from build123d import *

# Parameters (mm, degrees)
BASE_EXTRUDE_THIN_DEPTH = 142.875
CUT_CNR_DEPTH           = 7.35
CUT_CNR_DEPTH_BACK      = 50.276
HOLE_FLG_D              = 16.764
HOLE_TOP_D              = 13.49375
HOLE_TOP_DEPTH          = 25.4


with BuildPart() as part:
    # Sketch1 → Base-Extrude-Thin (new body)
    with BuildSketch(Plane.XY):
        with BuildLine():
            Line((-228.6, 0), (-6.35, 0))
            ThreePointArc((-6.35, 0), (-1.859871939, -1.859871939), (0, -6.35))
            Line((0, -6.35), (0, -49.276))
            Line((0, -49.276), (6.35, -49.276))
            Line((6.35, -49.276), (6.35, -6.35))
            ThreePointArc((6.35, -6.35), (2.630256121, 2.630256121), (-6.35, 6.35))
            Line((-6.35, 6.35), (-228.6, 6.35))
            Line((-228.6, 6.35), (-228.6, 0))
        make_face()
    extrude(amount=BASE_EXTRUDE_THIN_DEPTH)

    # Sketch2 → Cut cnr (cut, two sides)
    with BuildSketch(Plane(origin=(0, 0, 0), x_dir=(1, 0, 0), z_dir=(0, 1, 0))) as cut_cnr_sk:
        Polygon((-714.082135383, 156.243851855), (-228.6, -50.8), (-12.7, -142.875), (472.782135383, -349.918851855), (58.694431674, -1320.883122621), (-1128.169839092, -814.720418912), align=None)
    extrude(amount=CUT_CNR_DEPTH, mode=Mode.SUBTRACT)
    extrude(cut_cnr_sk.sketch, amount=-CUT_CNR_DEPTH_BACK, mode=Mode.SUBTRACT)

    # Hole-flg (through all)
    with Locations(Plane(origin=(6.35, 0, 0), x_dir=(0, 0, -1), z_dir=(1, 0, 0))):
        with Locations((-120.65, -26.924), (-22.225, -26.924)):
            Hole(HOLE_FLG_D / 2)

    # Hole-top
    with Locations(Plane(origin=(0, 6.35, 0), x_dir=(-1, 0, 0), z_dir=(0, 1, 0))):
        with Locations((203.2, 31.75), (133.35, 31.75)):
            Hole(HOLE_TOP_D / 2, depth=HOLE_TOP_DEPTH)


solid = part.part
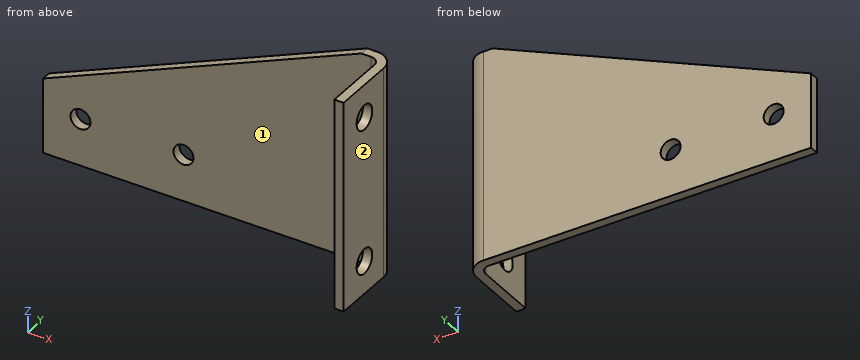
Could you check a few things on this model? Use its own coordinates, in mm. Face numbers are marked on the shaded views. A direction names the side the tool comes from. Coordinates: 2 decimals unless noted, no trailing zeros. Order: outer loops, then holes, each group sorted by start corner. A loop starts at its lowest first (then second) coordinate and runs counter-clockwise, first axis right, second up.
Q1. Suppose I cut it at A-A on x = -133.35. Please give me the cut outline in (y, z).
Q2. Please list where these lines run through material, in increasing order: L1, parallel to Y at x = -34, z = 112.5; L2, parallel to X at y = 3, z = 31.
Q3. Suppose I cut it at D-D on y = -16. Please give me the cut outline in (x, z) (3 decimals), and give its area (3 significant figures).
Q4. Which directions (+Z, -Z, +X, -X, +Y, -Y) give clear straight access to the entire face, cutting with the end or side of a thin tool? Please do the marked faces 1 and 2.
Q5. Suppose I cut it at C-C on z = 41. Please give me the cut outline in (x, y).
Q6. Will these pins go through, and if not, where does the flat tip stop? pin 1 (6 mm diameter, centred on y = -0.5, z = 92, fed in from -X); pin 2 (2 mm diameter, centred on y = -36.5, z = 97.5, fed in from -X); pin 3 (3 mm diameter, centred on y = -1.5, z = 76, fed in from +X); pin 4 (12 mm diameter, centred on x = -203.2, z = 31.75, fed in from +Y).
Q7. Suppose I cut it at B-B on z = 19.5. Please give me the cut outline in (x, y).
Answer:
1. outline: (0, 0) - (6.35, 0) - (6.35, 25) - (0, 25) - close; (0, 38.5) - (6.35, 38.5) - (6.35, 91.42) - (0, 91.42) - close
2. L1: y = 0 to 6.35
2. L2: x = -228.6 to -209.91, -196.49 to -140.06, -126.64 to 2.24
3. outline: (0, 0) - (6.35, 0) - (6.35, 142.875) - (0, 142.875) - close
3. area: 907 mm2
4. face 1: +Z, -Z, -X, -Y
4. face 2: +Z, -Z, +X, +Y, -Y
5. outline: (-228.6, 0) - (-6.35, 0) arc R6.35 cw to (0, -6.35) - (0, -49.28) - (6.35, -49.28) - (6.35, -6.35) arc R12.7 ccw to (-6.35, 6.35) - (-228.6, 6.35) - close
6. pin 1: stops at x = -138.93
6. pin 2: stops at x = 0
6. pin 3: stops at x = 5.9
6. pin 4: passes through
7. outline: (-228.6, 0) - (-6.35, 0) arc R6.35 cw to (0, -6.35) - (0, -19) - (6.35, -19) - (6.35, -6.35) arc R12.7 ccw to (-6.35, 6.35) - (-228.6, 6.35) - close; (0, -49.28) - (6.35, -49.28) - (6.35, -34.85) - (0, -34.85) - close
